from build123d import *

# Parameters (mm, degrees)
SKETCH1_R           = 1.778
SKETCH1_R_2         = 1.2065
BOSS_EXTRUDE1_DEPTH = 57.15
CUT_EXTRUDE1_DEPTH  = 53.594
CUT_EXTRUDE2_DEPTH  = 8.128
FILLET2_R           = 1.27
FILLET3_R           = 1.27
CUT_EXTRUDE3_DEPTH  = 3.048


with BuildPart() as part:
    # Sketch1 → Boss-Extrude1 (new body)
    with BuildSketch(Plane.XY):
        with BuildLine():
            Line((-9.0932, 13.8049), (9.0932, 13.8049))
            ThreePointArc((9.0932, 13.8049), (13.583328061, 11.945028061), (15.4432, 7.4549))
            Line((15.4432, 7.4549), (15.4432, -7.4549))
            ThreePointArc((15.4432, -7.4549), (13.583328061, -11.945028061), (9.0932, -13.8049))
            Line((9.0932, -13.8049), (-9.0932, -13.8049))
            ThreePointArc((-9.0932, -13.8049), (-13.583328061, -11.945028061), (-15.4432, -7.4549))
            Line((-15.4432, -7.4549), (-15.4432, 7.4549))
            ThreePointArc((-15.4432, 7.4549), (-13.583328061, 11.945028061), (-9.0932, 13.8049))
        make_face()
        with Locations((-8.0772, 7.7851)):
            Circle(SKETCH1_R, mode=Mode.SUBTRACT)
        with Locations(Location((6.834359756, -8.896092883, 0), (0, 0, 180))):
            Circle(SKETCH1_R, mode=Mode.SUBTRACT)
        with Locations((2.065458908, 2.065458908)):
            Circle(SKETCH1_R_2, mode=Mode.SUBTRACT)
        with Locations((2.065458908, -2.065458908)):
            Circle(SKETCH1_R_2, mode=Mode.SUBTRACT)
        with Locations((-2.065458908, -2.065458908)):
            Circle(SKETCH1_R_2, mode=Mode.SUBTRACT)
        with Locations((-2.065458908, 2.065458908)):
            Circle(SKETCH1_R_2, mode=Mode.SUBTRACT)
    extrude(amount=BOSS_EXTRUDE1_DEPTH)

    # Sketch2 → Cut-Extrude1 (cut)
    with BuildSketch(Plane(origin=(0, 0, 1.778), x_dir=(-1, 0, 0), z_dir=(0, 0, -1))):
        with BuildLine():
            Line((-12.315875439, 12.926358947), (-12.315875439, 13.8049))
            Line((-12.315875439, 13.8049), (-0.635, 13.8049))
            Line((-0.635, 13.8049), (-0.635, 0.4699))
            Line((-0.635, 0.4699), (-14.1732, 0.4699))
            Line((-14.1732, 0.4699), (-14.1732, 7.4549))
            ThreePointArc((-14.1732, 7.4549), (-13.696211827, 10.343953372), (-12.315875439, 12.926358947))
        make_face()
        with BuildLine():
            Line((14.1732, 0.4699), (0.635, 0.4699))
            Line((0.635, 0.4699), (0.635, 13.8049))
            Line((0.635, 13.8049), (12.315875439, 13.8049))
            Line((12.315875439, 13.8049), (12.315875439, 12.926358947))
            ThreePointArc((12.315875439, 12.926358947), (13.696211827, 10.343953372), (14.1732, 7.4549))
            Line((14.1732, 7.4549), (14.1732, 0.4699))
        make_face()
        with BuildLine():
            Line((-14.1732, -7.4549), (-14.1732, -0.4699))
            Line((-14.1732, -0.4699), (-0.635, -0.4699))
            Line((-0.635, -0.4699), (-0.635, -13.8049))
            Line((-0.635, -13.8049), (-12.315875439, -13.8049))
            Line((-12.315875439, -13.8049), (-12.315875439, -12.926358947))
            ThreePointArc((-12.315875439, -12.926358947), (-13.696211827, -10.343953372), (-14.1732, -7.4549))
        make_face()
        with BuildLine():
            Line((14.1732, -0.4699), (0.635, -0.4699))
            Line((0.635, -0.4699), (0.635, -13.8049))
            Line((0.635, -13.8049), (12.315875439, -13.8049))
            Line((12.315875439, -13.8049), (12.315875439, -12.926358947))
            ThreePointArc((12.315875439, -12.926358947), (13.696211827, -10.343953372), (14.1732, -7.4549))
            Line((14.1732, -7.4549), (14.1732, -0.4699))
        make_face()
    extrude(amount=-CUT_EXTRUDE1_DEPTH, mode=Mode.SUBTRACT)

    # Sketch3 → Cut-Extrude2 (cut)
    with BuildSketch(Plane.ZY.offset(15.4432)):
        with BuildLine():
            Line((1.778, 12.926358947), (1.778, 5.207))
            ThreePointArc((1.778, 5.207), (1.963987194, 4.757987194), (2.413, 4.572))
            Line((2.413, 4.572), (4.191, 4.572))
            ThreePointArc((4.191, 4.572), (4.640012806, 4.757987194), (4.826, 5.207))
            Line((4.826, 5.207), (4.826, 12.926358947))
            Line((4.826, 12.926358947), (1.778, 12.926358947))
        make_face()
        with BuildLine():
            Line((54.737, 4.572), (52.959, 4.572))
            ThreePointArc((52.959, 4.572), (52.509987194, 4.757987194), (52.324, 5.207))
            Line((52.324, 5.207), (52.324, 12.926358947))
            Line((52.324, 12.926358947), (55.372, 12.926358947))
            Line((55.372, 12.926358947), (55.372, 5.207))
            ThreePointArc((55.372, 5.207), (55.186012806, 4.757987194), (54.737, 4.572))
        make_face()
        with BuildLine():
            Line((2.413, -4.572), (4.191, -4.572))
            ThreePointArc((4.191, -4.572), (4.640012806, -4.757987194), (4.826, -5.207))
            Line((4.826, -5.207), (4.826, -12.926358947))
            Line((4.826, -12.926358947), (1.778, -12.926358947))
            Line((1.778, -12.926358947), (1.778, -5.207))
            ThreePointArc((1.778, -5.207), (1.963987194, -4.757987194), (2.413, -4.572))
        make_face()
        with BuildLine():
            Line((54.737, -4.572), (52.959, -4.572))
            ThreePointArc((52.959, -4.572), (52.509987194, -4.757987194), (52.324, -5.207))
            Line((52.324, -5.207), (52.324, -12.926358947))
            Line((52.324, -12.926358947), (55.372, -12.926358947))
            Line((55.372, -12.926358947), (55.372, -5.207))
            ThreePointArc((55.372, -5.207), (55.186012806, -4.757987194), (54.737, -4.572))
        make_face()
        with BuildLine():
            Line((19.685, 12.926358947), (37.465, 12.926358947))
            Line((37.465, 12.926358947), (37.465, 5.207))
            ThreePointArc((37.465, 5.207), (37.279012806, 4.757987194), (36.83, 4.572))
            Line((36.83, 4.572), (20.32, 4.572))
            ThreePointArc((20.32, 4.572), (19.870987194, 4.757987194), (19.685, 5.207))
            Line((19.685, 5.207), (19.685, 12.926358947))
        make_face()
        with BuildLine():
            Line((37.465, -12.926358947), (37.465, -5.207))
            ThreePointArc((37.465, -5.207), (37.279012806, -4.757987194), (36.83, -4.572))
            Line((36.83, -4.572), (20.32, -4.572))
            ThreePointArc((20.32, -4.572), (19.870987194, -4.757987194), (19.685, -5.207))
            Line((19.685, -5.207), (19.685, -12.926358947))
            Line((19.685, -12.926358947), (37.465, -12.926358947))
        make_face()
    cut_extrude2 = extrude(amount=-CUT_EXTRUDE2_DEPTH, mode=Mode.SUBTRACT)

    # Mirror1: Cut-Extrude2 across plane
    add(cut_extrude2.mirror(Plane(origin=(0, 0, 0), x_dir=(0, 0, 1), z_dir=(1, 0, 0))), mode=Mode.SUBTRACT)

    # Fillet2
    fillet2_edges = [part.edges().sort_by_distance(p)[0] for p in [
        (-13.583328061, 11.945028061, 57.15),
        (-15.4432, 0, 57.15),
        (-13.583328061, -11.945028061, 57.15),
        (0, -13.8049, 57.15),
        (13.583328061, -11.945028061, 57.15),
        (15.4432, 0, 57.15),
        (13.583328061, 11.945028061, 57.15),
        (0, 13.8049, 57.15),
    ]]
    fillet(fillet2_edges, radius=FILLET2_R)

    # Fillet3
    fillet3_edges = [part.edges().sort_by_distance(p)[0] for p in [
        (0, 13.8049, 0),
        (13.583328061, 11.945028061, 0),
        (15.4432, 0, 0),
        (13.583328061, -11.945028061, 0),
        (0, -13.8049, 0),
        (-13.583328061, -11.945028061, 0),
        (-15.4432, 0, 0),
        (-13.583328061, 11.945028061, 0),
    ]]
    fillet(fillet3_edges, radius=FILLET3_R)

    # Sketch4 → Cut-Extrude3 (cut)
    with BuildSketch(Plane(origin=(0.635, 0, 0), x_dir=(0, 0, -1), z_dir=(1, 0, 0))):
        with BuildLine():
            Line((-20.917407266, 4.572), (-36.232592734, 4.572))
            ThreePointArc((-36.232592734, 4.572), (-36.814131461, 4.63946836), (-37.364776122, 4.838289206))
            Line((-37.364776122, 4.838289206), (-55.372, 13.8049))
            Line((-55.372, 13.8049), (-1.778, 13.8049))
            Line((-1.778, 13.8049), (-19.785223878, 4.838289206))
            ThreePointArc((-19.785223878, 4.838289206), (-20.335868539, 4.63946836), (-20.917407266, 4.572))
        make_face()
        with BuildLine():
            Line((-55.372, -13.8049), (-1.778, -13.8049))
            Line((-1.778, -13.8049), (-19.785223878, -4.838289206))
            ThreePointArc((-19.785223878, -4.838289206), (-20.335868539, -4.63946836), (-20.917407266, -4.572))
            Line((-20.917407266, -4.572), (-36.232592734, -4.572))
            ThreePointArc((-36.232592734, -4.572), (-36.814131461, -4.63946836), (-37.364776122, -4.838289206))
            Line((-37.364776122, -4.838289206), (-55.372, -13.8049))
        make_face()
    extrude(amount=-CUT_EXTRUDE3_DEPTH, mode=Mode.SUBTRACT)


solid = part.part
Could you check a few things on this model? Use its own coordinates, in mm. A direction names the side the tool comes from. Give positions to 0.01 mm unless a question says otherwise; leave off trailing zeros. Write each loop counter-clockwise with the first axis right and the second up, starting at its lowest first coordinate (ties: lowest second). Pieces come first, ordered by that corner, then holes. Notation, with made-up numbers: (34.25, 88.5) - (82.25, 88.5) arc R34 ccw to (82.25, 123.5) - close; hole circle Ø5 at (-13.75, 6). An arc over 180 degrees is marked (long way). Use CSV: the item, a comma, the result in double quotes. Start each with the question number.
Item 1: I want a section at C-C, the plane y = 11. Give the number of separate pieces and of enclosed holes in the cut face, then the cut area to 3 significant figures.
Item 2: I want a section at A-A, the plane x = -4. Please give me the cut outline in (y, z), then the cut area to 3 significant figures.
Item 3: I'm going to push flat-ended pins straight in: pin 1 (4 mm diameter, centred on x = -9.5, z = 24, fed in from -Y); pin 2 (10 mm diameter, centred on x = -10, z = 31, fed in from +Y); pin 3 (0.6 mm diameter, centred on x = 15, z = 54, fed in from -Y). Where does each tip first touch, or does it pass through?
Item 4: If I drill on line 1 along X through (y, z) = (1, 34.5) (3 decimals); line 2 along Z through (x, y) = (-1, 4); line 3 along Y through (x, z) = (1.5, 14), over which ranges is the centre line in solid material (lowest first)?
Item 5: I want a section at D-D, the plane z = 49.5. Please give me the cut outline in (x, y) (3 decimals).
Item 6: If we mould it in two halves opening along X, with no side actions, what happens to faces 6 (the face through (14.4, -8.5, 52.324)), 7 (the face through (0.01, 9.38, 10.66)), 8 (the face through (14.58, 10.65, 12.15))? For each: pulls with the +X half, pulls with the -X half, needs draft (parallel to the pull), parting line crosses it, or undercut.
Item 7: For faces 1 (the face through (-8.1, 5.7, 1.778)), 2 (the face through (13.71, 10.3, 12.15)), 3 (the face through (-0.635, -4, 28)), 4 (the face through (14.4, 8.5, 19.685)), 5 (the face through (0.01, -4.64, 20.33)), which set-ups out of +Z, -Z, +X, -X, +Y, -Y let a thin tool reach every point of the face, with its end or its side?
Item 8: I want a section at B-B, the plane z = 32.5. Please give me the cut outline in (x, y) (3 decimals), then the cut area to 3 significant figures.
Findings:
1,separate pieces,"6"
1,enclosed holes,"0"
1,area,"169 mm2"
2,outline,"(-13.8, 1.27) arc R1.27 ccw to (-12.53, 0) - (12.53, 0) arc R1.27 ccw to (13.8, 1.27) - (13.8, 1.78) - (0.47, 1.78) - (0.47, 55.37) - (13.8, 55.37) - (13.8, 55.88) arc R1.27 ccw to (12.53, 57.15) - (-12.53, 57.15) arc R1.27 ccw to (-13.8, 55.88) - (-13.8, 55.37) - (-0.47, 55.37) - (-0.47, 1.78) - (-13.8, 1.78) - close"
2,area,"147 mm2"
3,pin 1,"stops at y = -0.47"
3,pin 2,"stops at y = 4.57"
3,pin 3,"stops at y = -4.57"
4,line 1,"x = -15.443 to -14.173, -0.635 to 0.635, 14.173 to 15.443"
4,line 2,"z = 0 to 1.78, 55.37 to 57.15"
4,line 3,"y = -0.47 to 0.47"
5,outline,"(-15.443, -7.455) arc R6.35 ccw to (-12.316, -12.926) arc R8.988 cw to (-14.173, -7.455) - (-14.173, -0.47) - (-0.635, -0.47) - (-0.635, -10.881) - (0.635, -10.881) - (0.635, -0.47) - (14.173, -0.47) - (14.173, -7.455) arc R8.988 cw to (12.316, -12.926) arc R6.35 ccw to (15.443, -7.455) - (15.443, 7.455) arc R6.35 ccw to (12.316, 12.926) arc R8.988 cw to (14.173, 7.455) - (14.173, 0.47) - (0.635, 0.47) - (0.635, 10.881) - (-0.635, 10.881) - (-0.635, 0.47) - (-14.173, 0.47) - (-14.173, 7.455) arc R8.988 cw to (-12.316, 12.926) arc R6.35 ccw to (-15.443, 7.455) - close"
6,face 6,"needs draft"
6,face 7,"undercut"
6,face 8,"pulls with the +X half"
7,face 1,"+Y"
7,face 2,"none"
7,face 3,"-Y"
7,face 4,"+X, -X, +Y"
7,face 5,"+X, -X, -Y"
8,outline,"(-15.443, -4.572) - (-14.173, -4.572) - (-14.173, -0.47) - (-0.635, -0.47) - (-0.635, -4.572) - (0.635, -4.572) - (0.635, -0.47) - (14.173, -0.47) - (14.173, -4.572) - (15.443, -4.572) - (15.443, 4.572) - (14.173, 4.572) - (14.173, 0.47) - (0.635, 0.47) - (0.635, 4.572) - (-0.635, 4.572) - (-0.635, 0.47) - (-14.173, 0.47) - (-14.173, 4.572) - (-15.443, 4.572) - close"
8,area,"60.3 mm2"
